from build123d import *

# Parameters (mm, degrees)
CONEREVOLVE_ANGLE                = 90
CONEREVOLVE_OTHER_WAY_ANGLE      = 90
CONE_EDGE_BOSS_EXTRUDE15_DEPTH   = 2.2
MOUNTING_HOLE_CUT_EXTRUDE6_REACH = 61.483
SKETCH90_R                       = 0.76
REINFORCINGSPAR_DEPTH            = 2
REINFORCINGSPAR_DEPTH_BACK       = 2
SKETCH94_W                       = 4
SKETCH94_H                       = 9.744950827
CUT_EXTRUDE1_DEPTH               = 6
FILLET2_SIZE                     = 2
SKETCH98_R                       = 0.762
CUT_EXTRUDE2_DEPTH               = 8


with BuildPart() as part:
    # Sketch88 → ConeRevolve (revolve)
    with BuildSketch(Plane(origin=(50.074313091, 0, 0), x_dir=(1, 0, 0), z_dir=(0, 0, 1))):
        Polygon((-82.2978509, 33.039348741), (-59.278041261, 3.039348741), (-60.538513675, 3.039348741), (-83.558323314, 33.039348741), align=None)
    revolve(axis=Axis((-2.2, -0.345734695, 0), (0, 1, 0)), revolution_arc=CONEREVOLVE_ANGLE)

    # Sketch88 → ConeRevolve other way (revolve)
    with BuildSketch(Plane(origin=(50.074313091, 0, 0), x_dir=(1, 0, 0), z_dir=(0, 0, 1))):
        Polygon((-82.2978509, 33.039348741), (-59.278041261, 3.039348741), (-60.538513675, 3.039348741), (-83.558323314, 33.039348741), align=None)
    revolve(axis=Axis((-2.2, -0.345734695, 0), (0, -1, 0)), revolution_arc=CONEREVOLVE_OTHER_WAY_ANGLE)

    # Sketch89 → Cone-Edge-Boss-Extrude15 (add)
    with BuildSketch(Plane(origin=(-2.2, 0, 0), x_dir=(0, 0, -1), z_dir=(1, 0, 0))):
        Polygon((-7.00372817, 3.039348741), (-8.264200584, 3.039348741), (-31.284010223, 33.039348741), (-30.023537809, 33.039348741), align=None)
        Polygon((8.264200584, 3.039348741), (7.00372817, 3.039348741), (30.023537809, 33.039348741), (31.284010223, 33.039348741), align=None)
    extrude(amount=CONE_EDGE_BOSS_EXTRUDE15_DEPTH)

    # Cone-Edge-Mirror: part across plane


with BuildPart() as part_1:
    add(part.part)
    add(part.part.mirror(Plane(origin=(0, 0, 0), x_dir=(0, 0, 1), z_dir=(1, 0, 0))))

    # Sketch90 → Mounting-Hole-Cut-Extrude6 (cut, up to next)
    with BuildSketch(Plane(origin=(0, -2.256187259, 2.940320481), x_dir=(1, 0, 0), z_dir=(2.7745173069220206e-15, -0.6087614290087164, 0.7933533402912384)), mode=Mode.PRIVATE) as mounting_hole_cut_extrude6_sk1:
        with Locations(Location((0, 15.169995435, 0), (0, 0, 90))):
            Circle(SKETCH90_R)
    mounting_hole_cut_extrude6_tool1 = extrude(mounting_hole_cut_extrude6_sk1.sketch, amount=MOUNTING_HOLE_CUT_EXTRUDE6_REACH, mode=Mode.PRIVATE) & part_1.part
    mounting_hole_cut_extrude6 = mounting_hole_cut_extrude6_tool1.solids().sort_by_distance((0, 9.778979, 12.175229))[0]
    add(mounting_hole_cut_extrude6, mode=Mode.SUBTRACT)

    # Mirror1: Mounting-Hole-Cut-Extrude6 across plane
    add(mounting_hole_cut_extrude6.mirror(Plane.XY), mode=Mode.SUBTRACT)

    # Sketch92 → ReinforcingSpar (add, two sides: drawn at the far end of the back side and taken through both)
    with BuildSketch(Plane(origin=(0, 0, 4.051072987), x_dir=(0, 0, -1), z_dir=(1, 0, 0)).offset(-REINFORCINGSPAR_DEPTH_BACK)):
        Polygon((-11.203976186, 33.039348741), (-27.232937236, 33.039348741), (-11.203976186, 12.15), align=None)
        Polygon((19.30612216, 33.039348741), (35.33508321, 33.039348741), (19.30612216, 12.15), align=None)
    extrude(amount=REINFORCINGSPAR_DEPTH + REINFORCINGSPAR_DEPTH_BACK)

    # Sketch94 → Cut-Extrude1 (cut)
    with BuildSketch(Plane(origin=(0, 33.039348741, 0), x_dir=(1, 0, 0), z_dir=(0, 1, 0))):
        with Locations((0, 20.127524587)):
            Rectangle(SKETCH94_W, SKETCH94_H)
        with Locations((0, -20.127524587)):
            Rectangle(SKETCH94_W, SKETCH94_H)
    extrude(amount=-CUT_EXTRUDE1_DEPTH, mode=Mode.SUBTRACT)

    # Fillet2
    # a fillet whose section is not a circle: 2 mm, written as the material it adds along each edge
    with BuildSketch(Plane(origin=(-2, 27.039348741, -25), x_dir=(0, 1, 0), z_dir=(1, 0, 0))) as fillet2_piece_1:
        with BuildLine():
            add(Edge.make_bspline([(FILLET2_SIZE, 0), (FILLET2_SIZE * 0.831801948466, 0), (FILLET2_SIZE * 0.663603896932, 0), (FILLET2_SIZE * 0.292893218813, FILLET2_SIZE * 0.0716919198361), (FILLET2_SIZE * 0.0716919198361, FILLET2_SIZE * 0.292893218813), (0, FILLET2_SIZE * 0.663603896932), (0, FILLET2_SIZE * 0.831801948466), (0, FILLET2_SIZE)], knots=[0, 0, 0, 0, 0, 0, 0.5, 0.5, 1, 1, 1, 1, 1, 1], degree=5))
            Line((0, FILLET2_SIZE), (-FILLET2_SIZE * 0.02, FILLET2_SIZE))
            Line((-FILLET2_SIZE * 0.02, FILLET2_SIZE), (-FILLET2_SIZE * 0.02, -FILLET2_SIZE * 0.02))
            Line((-FILLET2_SIZE * 0.02, -FILLET2_SIZE * 0.02), (FILLET2_SIZE, -FILLET2_SIZE * 0.02))
            Line((FILLET2_SIZE, -FILLET2_SIZE * 0.02), (FILLET2_SIZE, 0))
        make_face()
    extrude(amount=4)
    with BuildSketch(Plane(origin=(-2, 27.039348741, 25), x_dir=(0, 1, 0), z_dir=(1, 0, 0))) as fillet2_piece_2:
        with BuildLine():
            add(Edge.make_bspline([(FILLET2_SIZE, 0), (FILLET2_SIZE * 0.831801948466, 0), (FILLET2_SIZE * 0.663603896932, 0), (FILLET2_SIZE * 0.292893218813, -FILLET2_SIZE * 0.0716919198361), (FILLET2_SIZE * 0.0716919198361, -FILLET2_SIZE * 0.292893218813), (0, -FILLET2_SIZE * 0.663603896932), (0, -FILLET2_SIZE * 0.831801948466), (0, -FILLET2_SIZE)], knots=[0, 0, 0, 0, 0, 0, 0.5, 0.5, 1, 1, 1, 1, 1, 1], degree=5))
            Line((0, -FILLET2_SIZE), (-FILLET2_SIZE * 0.02, -FILLET2_SIZE))
            Line((-FILLET2_SIZE * 0.02, -FILLET2_SIZE), (-FILLET2_SIZE * 0.02, FILLET2_SIZE * 0.02))
            Line((-FILLET2_SIZE * 0.02, FILLET2_SIZE * 0.02), (FILLET2_SIZE, FILLET2_SIZE * 0.02))
            Line((FILLET2_SIZE, FILLET2_SIZE * 0.02), (FILLET2_SIZE, 0))
        make_face()
    extrude(amount=4)

    # Sketch98 → Cut-Extrude2 (cut)
    with BuildSketch(Plane(origin=(0, 33.039348741, 0), x_dir=(1, 0, 0), z_dir=(0, 1, 0))):
        with Locations(Location((0, -22.2, 0), (0, 0, 270))):
            Circle(SKETCH98_R)
        with Locations(Location((0, 22.2, 0), (0, 0, 270))):
            Circle(SKETCH98_R)
    extrude(amount=-CUT_EXTRUDE2_DEPTH, mode=Mode.SUBTRACT)


solid = part_1.part
Geometry check sheet. Reference: the model listing, model coordinates, mm. A direction names the side the tool comes from. Round coordinates to 2 decimals unless told otherwise and drop trailing zeros. Order: outer loops, then holes, each group sorted by start corner. A loop starts at its lowest first (then second) coordinate and runs counter-clockwise, first axis right, second up. Notation, with made-up numbers: M -4.75,77 L 27.25,77 A27 cw 27.25,111 Z; hole C -7.5,65 d2. An arc over 180 degrees is marked long. Answer in a Markdown table with one row per item. Add a question column.
Item 1: Sectioned sample at B-B, the plane y = 31. Enter the section's corners in (x, z), plus the area to 3 significant figures.
Item 2: Depth check by flat-ended pin: pin 1 Ø12 at (y, z) = (28, 20) entering from +X; pin 2 Ø5 at (y, z) = (18.5, -1) entering from -X; pin 3 Ø10 at (y, z) = (18, -8) entering from +X. Enter the tip coordinate at first touch or a pass-through.
Item 3: Sectioned sample at A-A, the plane y = 23.5. Enter the section's corners in (x, z), plus the area to 3 significant figures.
Item 4: Draft check along Z on faces 1 (the face through (0.229, 26.053, -21.473)), 2 (the face through (-0.031, 18.249, 19.935)), 3 (the face through (19.573, 14.916, 0.382)). Enter one of: released by +Z, released by -Z, zero draft, split by the parting line, or undercut.
Item 5: Material ranges on L1, parallel to X at y = 26.5, z = -22.2; L2, parallel to X at y = 25.55, z = -22.2; L3, parallel to Z at x = 0, y = 25, recorded low to high. Write a range as [from, to].
Item 6: Set-up check for faces 4 (the face through (0.031, 18.249, -19.935)), 5 (the face through (2, 24, 20)): record each of +Z, -Z, +X, -X, +Y, -Y from which the full face is reachable in a straight line by a thin tool's end or side.
Filled in:
| question | item | result |
|---|---|---|
| 1 | outline | M -2.2,-29.72 L 2.2,-29.72 A29.72 ccw 2.2,29.72 L -2.2,29.72 A29.72 ccw Z; hole M -2.2,-28.46 L -2,-28.46 L -2,-25 L 2,-25 L 2,-28.46 L 2.2,-28.46 A28.46 ccw 2.2,28.46 L 2,28.46 L 2,25 L -2,25 L -2,28.46 L -2.2,28.46 A28.46 ccw Z |
| 1 | area | 269 mm² |
| 2 | pin 1 | stops at x = 28.63 |
| 2 | pin 2 | stops at x = -24.23 |
| 2 | pin 3 | stops at x = 24.69 |
| 3 | outline | M -2.2,-23.96 L 2.2,-23.96 A23.96 ccw 2.2,23.96 L -2.2,23.96 A23.96 ccw Z; hole M -2.2,-22.7 L -2,-22.7 L -2,-15.26 L 2,-15.26 L 2,-22.7 L 2.2,-22.7 A22.7 ccw 2.2,22.7 L 2,22.7 L 2,15.26 L -2,15.26 L -2,22.7 L -2.2,22.7 A22.7 ccw Z |
| 3 | area | 255 mm² |
| 4 | face 1 | undercut |
| 4 | face 2 | released by +Z |
| 4 | face 3 | split by the parting line |
| 5 | L1 | x = [-16.24, -13.71], [-2, -0.76], [0.76, 2], [13.71, 16.24] |
| 5 | L2 | x = [-14.82, -12.02], [-2, -0.76], [0.76, 2], [12.02, 14.82] |
| 5 | L3 | z = [-25.12, -15.26], [15.26, 25.12] |
| 6 | face 4 | -Z, +X, -X, -Y |
| 6 | face 5 | +Y |
